Read the model definition and answer for the solid it produces. Units are mm, in the model's axes. Face numbers are marked on the shaded views. A direction names the side the tool comes from. Coordinates: 2 decimals unless noted, no trailing zeros. Loops run counter-clockwise (first coordinate to the right, second up) from the corner with the lowest first, then second, coordinate; pieces in that order, holes last. Notation, with made-up numbers: (-14, -8) -> (4, -8) arc R16 ccw to (4, 0) -> close; hole circle Ø1 at (75, 88.25). An arc over 180 degrees is marked (long way). Answer as a JSON object with one key per item and string values. Group by question number.
Q1. The part is cut by section C-C on y = 34. Write down the section's boundary in (x, z), and give its area (3 significant figures).
Q2. The part is cut by section B-B on z = 19.05. Write down the section's boundary in (x, y) (3 decimals), and give its area (3 significant figures).
Q3. The part is cut by section D-D on x = 26.5. Write down the section's boundary in (y, z).
Q4. For the marked faces 1 and 2, determine the directions among +Z, -Z, +X, -X, +Y, -Y from which every point of the face is accessible in a straight line to the end or side of a thin tool.
Q5. Each of these flat-tipped pins is pushed along its axis until it touches: P1, Ø10, axis at x = -6, z = 17.5, coming from the +Y side; P2, Ø1.3, axis at y = 40.5, z = -34, coming from the +X side; P3, Ø0.8, axis at y = 40.5, z = -33.5, coming from the -X side. Where does it stop, or does it pass through?
Q6. The part is cut by section A-A on y = 17. Write down the section's boundary in (x, z).
Q7. Straight lines are drawn through the part: line 1 along Z through (x, y) = (12, 21.5); line 2 along X through (y, z) = (13.5, -1); line 3 along X through (y, z) = (15, -16.5). For each, find the intervals that lie inside material, in ascending order. Write a range as [from, to].
Q8. Determine the mould class of the marked faces 3, 4, 5 and 6 for opening direction Z: released by +Z, released by -Z, zero draft, split by the parting line, or undercut.
from build123d import *

# Parameters (mm, degrees)
SKETCH1_W            = 84.074
SKETCH1_H            = 77.724
BOSS_EXTRUDE1_DEPTH  = 5.08
SKETCH3_R            = 2.54
BOSS_EXTRUDE2_DEPTH  = 2.54
SKETCH19_W           = 12.7
SKETCH19_H           = 5.08
SKETCH19_W_2         = 10.16
BOSS_EXTRUDE7_DEPTH  = 33.02
FILLET2_R            = 10.16
SKETCH21_R           = 2.286
SKETCH21_W           = 7.112
SKETCH21_H           = 2.54
BOSS_EXTRUDE9_DEPTH  = 3.81
SKETCH22_W           = 12.446
SKETCH22_H           = 11.43
SKETCH22_W_2         = 9.779
SKETCH22_H_2         = 11.683309762
CUT_EXTRUDE10_DEPTH  = 5.08
SKETCH23_R           = 1.524
BOSS_EXTRUDE10_DEPTH = 3.81


with BuildPart() as part:
    # Sketch1 → Boss-Extrude1 (new body)
    with BuildSketch(Plane(origin=(0, 0, 0), x_dir=(1, 0, 0), z_dir=(0, 1, 0))):
        Rectangle(SKETCH1_W, SKETCH1_H)
    extrude(amount=BOSS_EXTRUDE1_DEPTH)

    # Sketch3 → Boss-Extrude2 (add)
    with BuildSketch(Plane(origin=(0, 5.08, 0), x_dir=(1, 0, 0), z_dir=(0, 1, 0))):
        with Locations((-19.939, 24.13)):
            Circle(SKETCH3_R)
        with Locations((-19.939, -24.13)):
            Circle(SKETCH3_R)
        with Locations((30.861, 8.89)):
            Circle(SKETCH3_R)
        with Locations((30.861, -19.05)):
            Circle(SKETCH3_R)
    extrude(amount=BOSS_EXTRUDE2_DEPTH)

    # Sketch19 → Boss-Extrude7 (add)
    with BuildSketch(Plane(origin=(0, 5.08, 0), x_dir=(1, 0, 0), z_dir=(0, 1, 0))):
        Polygon((-37.973, 34.798), (-42.037, 34.798), (-42.037, -34.798), (-37.973, -34.798), (-37.973, -29.718), (-37.973, 29.718), align=None)
        with Locations((-31.623, -32.258)):
            Rectangle(SKETCH19_W, SKETCH19_H)
        Polygon((42.037, -38.862), (42.037, 34.798), (37.973, 34.798), (37.973, 29.718), (37.973, -29.718), (37.973, -34.798), (37.973, -38.862), align=None)
        with Locations((32.893, 32.258)):
            Rectangle(SKETCH19_W_2, SKETCH19_H)
        Polygon((42.037, 38.862), (-42.037, 38.862), (-42.037, 34.798), (-37.973, 34.798), (-25.273, 34.798), (27.813, 34.798), (37.973, 34.798), (42.037, 34.798), align=None)
        with Locations((-31.623, 32.258)):
            Rectangle(SKETCH19_W, SKETCH19_H)
        Polygon((-37.973, -34.798), (-42.037, -34.798), (-42.037, -38.862), (37.973, -38.862), (37.973, -34.798), (27.813, -34.798), (-25.273, -34.798), align=None)
        with Locations((32.893, -32.258)):
            Rectangle(SKETCH19_W_2, SKETCH19_H)
    extrude(amount=BOSS_EXTRUDE7_DEPTH)

    # Fillet2
    fillet2_edges = [part.edges().sort_by_distance(p)[0] for p in [
        (42.037, 19.05, 38.862),
        (-42.037, 19.05, 38.862),
        (-42.037, 19.05, -38.862),
        (42.037, 19.05, -38.862),
    ]]
    fillet(fillet2_edges, radius=FILLET2_R)

    # Sketch21 → Boss-Extrude9 (add)
    with BuildSketch(Plane(origin=(0, 38.1, 0), x_dir=(1, 0, 0), z_dir=(0, 1, 0))):
        with Locations((32.893, 34.29)):
            Circle(SKETCH21_R)
        with Locations((-31.877, 33.782)):
            Rectangle(SKETCH21_W, SKETCH21_H)
    boss_extrude9 = extrude(amount=BOSS_EXTRUDE9_DEPTH)

    # Sketch22 → Cut-Extrude10 (cut)
    with BuildSketch(Plane.ZY.offset(42.037)):
        with Locations((-12.827, 14.986)):
            Rectangle(SKETCH22_W, SKETCH22_H)
        with Locations((17.2085, 15.112654881)):
            Rectangle(SKETCH22_W_2, SKETCH22_H_2)
    extrude(amount=-CUT_EXTRUDE10_DEPTH, mode=Mode.SUBTRACT)

    # Sketch23 → Boss-Extrude10 (add)
    with BuildSketch(Plane(origin=(0, 7.62, 0), x_dir=(1, 0, 0), z_dir=(0, 1, 0))):
        with Locations((-19.939, 24.13)):
            Circle(SKETCH23_R)
        with Locations((30.861, 8.89)):
            Circle(SKETCH23_R)
        with Locations((-19.939, -24.13)):
            Circle(SKETCH23_R)
        with Locations((30.861, -19.05)):
            Circle(SKETCH23_R)
    extrude(amount=BOSS_EXTRUDE10_DEPTH)

    # Mirror1: Boss-Extrude9 across plane
    add(boss_extrude9.mirror(Plane.XY))


solid = part.part
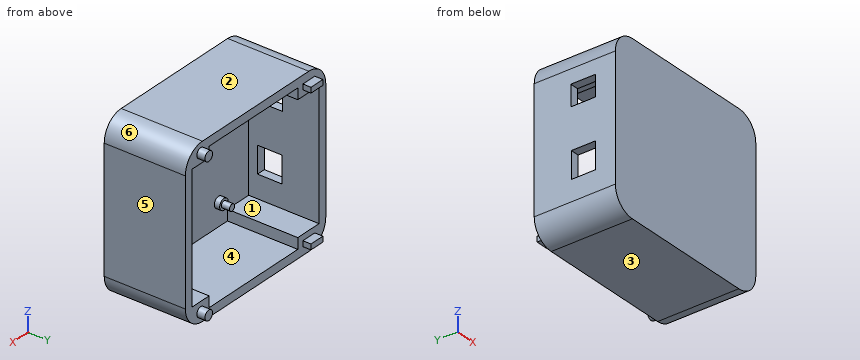
Final values:
{
 "1": {"outline": "(-42.04, -28.7) arc R10.16 ccw to (-31.88, -38.86) -> (31.88, -38.86) arc R10.16 ccw to (42.04, -28.7) -> (42.04, 28.7) arc R10.16 ccw to (31.88, 38.86) -> (-31.88, 38.86) arc R10.16 ccw to (-42.04, 28.7) -> close; hole (-37.97, -29.72) -> (-25.27, -29.72) -> (-25.27, -34.8) -> (27.81, -34.8) -> (27.81, -29.72) -> (37.97, -29.72) -> (37.97, 29.72) -> (27.81, 29.72) -> (27.81, 34.8) -> (-25.27, 34.8) -> (-25.27, 29.72) -> (-37.97, 29.72) -> close", "area": "1,390 mm2"},
 "2": {"outline": "(-42.037, 0) -> (42.037, 0) -> (42.037, 38.1) -> (37.973, 38.1) -> (37.973, 5.08) -> (33.401, 5.08) -> (33.401, 7.62) -> (32.385, 7.62) -> (32.385, 11.43) -> (29.337, 11.43) -> (29.337, 7.62) -> (28.321, 7.62) -> (28.321, 5.08) -> (-37.973, 5.08) -> (-37.973, 9.271) -> (-42.037, 9.271) -> close; (-42.037, 20.954) -> (-37.973, 20.954) -> (-37.973, 38.1) -> (-42.037, 38.1) -> close", "area": "673 mm2"},
 "3": {"outline": "(0, -38.86) -> (38.1, -38.86) -> (38.1, -34.8) -> (5.08, -34.8) -> (5.08, 34.8) -> (38.1, 34.8) -> (38.1, 38.86) -> (0, 38.86) -> close"},
 "4": {"face 1": "+Y", "face 2": "+Z, +X, -X, +Y, -Y"},
 "5": {"P1": "stops at y = 5.08", "P2": "stops at x = 35.18", "P3": "stops at x = -35.43"},
 "6": {"outline": "(-42.04, -28.7) arc R10.16 ccw to (-31.88, -38.86) -> (31.88, -38.86) arc R10.16 ccw to (42.04, -28.7) -> (42.04, 28.7) arc R10.16 ccw to (31.88, 38.86) -> (-31.88, 38.86) arc R10.16 ccw to (-42.04, 28.7) -> (-42.04, 22.1) -> (-37.97, 22.1) -> (-37.97, 29.72) -> (-25.27, 29.72) -> (-25.27, 34.8) -> (27.81, 34.8) -> (27.81, 29.72) -> (37.97, 29.72) -> (37.97, -29.72) -> (27.81, -29.72) -> (27.81, -34.8) -> (-25.27, -34.8) -> (-25.27, -29.72) -> (-37.97, -29.72) -> (-37.97, -19.05) -> (-42.04, -19.05) -> close; (-42.04, -6.6) -> (-37.97, -6.6) -> (-37.97, 12.32) -> (-42.04, 12.32) -> close"},
 "7": {"line 1": "z = [-38.86, -34.8], [34.8, 38.86]", "line 2": "x = [-42.04, -37.97], [37.97, 42.04]", "line 3": "x = [37.97, 42.04]"},
 "8": {"face 3": "released by -Z", "face 4": "undercut", "face 5": "zero draft", "face 6": "released by +Z"}
}
